Geometry check sheet. Reference: the model listing, model coordinates, mm. Round coordinates to 2 decimals unless told otherwise and drop trailing zeros. Order: outer loops, then holes, each group sorted by start corner. A loop starts at its lowest first (then second) coordinate and runs counter-clockwise, first axis right, second up. Notation, with made-up numbers: (60, 43.5) - (64, 43.5) arc R35 ccw to (64, 79.5) - close; hole circle Ø9 at (19.25, 34). An arc over 180 degrees is marked (long way). Use a Markdown table: item, result. Add a question column.
(1) Thickness scan on line 1 along Y through (x, z) = (0, 1.4); line 2 along X through (y, z) = (-4, 2.6); line 3 along Y through (x, z) = (30, 3.7). Record the ranges inside material, lowest first. Write a range as [from, to].
(2) Gauge pin test, flat ends, axial feed: P1, Ø1, axis at x = 7, y = -19, coming from the -Z side; P2, Ø1, axis at y = -11, z = 3, coming from the -X side; P3, Ø11.5, axis at x = -30, y = 0, coming from the +Z side. Record the tip position at first contact, or that the pin passes through.
(3) Section check B-B on x = 0. Record the boundary of the cut face in (y, z).
(4) Section check D-D on y = -18. Record the boundary of the cut face in (x, z).
(5) Section check A-A on y = 0. Record the boundary of the cut face in (x, z).
(6) Section check C-C on z = 2.6. Record the boundary of the cut face in (x, y).
(7) Mould release check, pull along X, two halves, no side actions. Record for faces 1 (the face through (-16.863, -12.93, 2.465)), 2 (the face through (15.46, 25.9, 2.54)), 3 (the face through (34.292, 1.352, 2.465)), 4 (the face through (-18, -12, 0)): released by +X, released by -X, zero draft, split by the parting line, or undercut.
```python
from build123d import *

# Parameters (mm, degrees)
ESQUISSE1_W        = 76.5
ESQUISSE1_H        = 56.5
ESQUISSE1_R        = 21.25
ESQUISSE1_R_2      = 4.5
BOSS_EXTRU_1_DEPTH = 5
CHANFREIN1_SIZE    = 22
CHANFREIN2_SIZE    = 22
CHANFREIN3_SIZE    = 22
CHANFREIN4_SIZE    = 22
CONG_2_R           = 30
CONG_3_R           = 30
CONG_4_R           = 30
CONG_5_R           = 30
CONG_6_R           = 12
CONG_7_R           = 12
CONG_8_R           = 12
CONG_9_R           = 12


with BuildPart() as part:
    # Esquisse1 → Boss.-Extru.1 (new body)
    with BuildSketch(Plane.XY):
        Rectangle(ESQUISSE1_W, ESQUISSE1_H)
        Circle(ESQUISSE1_R, mode=Mode.SUBTRACT)
        with Locations((30, 0)):
            Circle(ESQUISSE1_R_2, mode=Mode.SUBTRACT)
        with Locations((-30, 0)):
            Circle(ESQUISSE1_R_2, mode=Mode.SUBTRACT)
    extrude(amount=BOSS_EXTRU_1_DEPTH)

    # Chanfrein1
    chanfrein1_edges = [part.edges().sort_by_distance(p)[0] for p in [
        (38.25, 28.25, 2.5),
    ]]
    chamfer(chanfrein1_edges, length=CHANFREIN1_SIZE)

    # Chanfrein2
    chanfrein2_edges = [part.edges().sort_by_distance(p)[0] for p in [
        (-38.25, 28.25, 2.5),
    ]]
    chamfer(chanfrein2_edges, length=CHANFREIN2_SIZE)

    # Chanfrein3
    chanfrein3_edges = [part.edges().sort_by_distance(p)[0] for p in [
        (-38.25, -28.25, 2.5),
    ]]
    chamfer(chanfrein3_edges, length=CHANFREIN3_SIZE)

    # Chanfrein4
    chanfrein4_edges = [part.edges().sort_by_distance(p)[0] for p in [
        (38.25, -28.25, 2.5),
    ]]
    chamfer(chanfrein4_edges, length=CHANFREIN4_SIZE)

    # Congé2
    cong_2_edges = [part.edges().sort_by_distance(p)[0] for p in [
        (16.25, 28.25, 2.5),
    ]]
    fillet(cong_2_edges, radius=CONG_2_R)

    # Congé3
    cong_3_edges = [part.edges().sort_by_distance(p)[0] for p in [
        (-16.25, 28.25, 2.5),
    ]]
    fillet(cong_3_edges, radius=CONG_3_R)

    # Congé4
    cong_4_edges = [part.edges().sort_by_distance(p)[0] for p in [
        (16.25, -28.25, 2.5),
    ]]
    fillet(cong_4_edges, radius=CONG_4_R)

    # Congé5
    cong_5_edges = [part.edges().sort_by_distance(p)[0] for p in [
        (-16.25, -28.25, 2.5),
    ]]
    fillet(cong_5_edges, radius=CONG_5_R)

    # Congé6
    cong_6_edges = [part.edges().sort_by_distance(p)[0] for p in [
        (38.25, 6.25, 2.5),
    ]]
    fillet(cong_6_edges, radius=CONG_6_R)

    # Congé7
    cong_7_edges = [part.edges().sort_by_distance(p)[0] for p in [
        (38.25, -6.25, 2.5),
    ]]
    fillet(cong_7_edges, radius=CONG_7_R)

    # Congé8
    cong_8_edges = [part.edges().sort_by_distance(p)[0] for p in [
        (-38.25, 6.25, 2.5),
    ]]
    fillet(cong_8_edges, radius=CONG_8_R)

    # Congé9
    cong_9_edges = [part.edges().sort_by_distance(p)[0] for p in [
        (-38.25, -6.25, 2.5),
    ]]
    fillet(cong_9_edges, radius=CONG_9_R)


solid = part.part
```
Check sheet entries:
| question | item | result |
|---|---|---|
| 1 | line 1 | y = [-28.25, -21.25], [21.25, 28.25] |
| 1 | line 2 | x = [-37.94, -32.06], [-27.94, -20.87], [20.87, 27.94], [32.06, 37.94] |
| 1 | line 3 | y = [-14.5, -4.5], [4.5, 14.5] |
| 2 | P1 | passes through |
| 2 | P2 | stops at x = -34 |
| 2 | P3 | stops at z = 5 |
| 3 | outline | (-28.25, 0) - (-21.25, 0) - (-21.25, 5) - (-28.25, 5) - close; (21.25, 0) - (28.25, 0) - (28.25, 5) - (21.25, 5) - close |
| 4 | outline | (-26.5, 0) - (-11.29, 0) - (-11.29, 5) - (-26.5, 5) - close; (11.29, 0) - (26.5, 0) - (26.5, 5) - (11.29, 5) - close |
| 5 | outline | (-38.25, 0) - (-34.5, 0) - (-34.5, 5) - (-38.25, 5) - close; (-25.5, 0) - (-21.25, 0) - (-21.25, 5) - (-25.5, 5) - close; (21.25, 0) - (25.5, 0) - (25.5, 5) - (21.25, 5) - close; (34.5, 0) - (38.25, 0) - (38.25, 5) - (34.5, 5) - close |
| 6 | outline | (-38.25, -1.28) arc R12 ccw to (-34.74, -9.76) - (-25.04, -19.46) arc R30 ccw to (-3.82, -28.25) - (3.82, -28.25) arc R30 ccw to (25.04, -19.46) - (34.74, -9.76) arc R12 ccw to (38.25, -1.28) - (38.25, 1.28) arc R12 ccw to (34.74, 9.76) - (25.04, 19.46) arc R30 ccw to (3.82, 28.25) - (-3.82, 28.25) arc R30 ccw to (-25.04, 19.46) - (-34.74, 9.76) arc R12 ccw to (-38.25, 1.28) - close; hole circle Ø9 at (-30, 0); hole circle Ø42.5 at (0, 0); hole circle Ø9 at (30, 0) |
| 7 | face 1 | undercut |
| 7 | face 2 | released by +X |
| 7 | face 3 | undercut |
| 7 | face 4 | zero draft |
